Autodesk Inventor part; units mm, degrees
ref_plane "YZ Plane" through (0, 0, 0) normal (1, 0, 0) x (0, 1, 0)
ref_plane "XZ Plane" through (0, 0, 0) normal (0, 1, 0) x (-1, 0, 0)
ref_plane "XY Plane" through (0, 0, 0) normal (0, 0, 1) x (1, 0, 0)
sketch "Sketch1" plane through (0, 0, 0) normal (0, 0, 1) x (1, 0, 0)
  circle A0 centre (-1.3066, -22.8322) radius 2.3
  circle A1 centre (-1.3066, -22.8322) radius 4.5
  circle A2 centre (-1.1075, 27.1674) radius 2.5
  arc A3 (-5.8066, -22.8322) -> (-3.6075, 27.1674) centre (-152.4621, 8.6663) ccw
  arc A4 (1.3925, 27.1674) -> (3.1934, -22.8322) centre (150.0964, 7.4911) ccw
  point P0 (0, 0)
  point P1 (2.8463, -21.0992)
  point P2 (1.3093, 26.5276)
  point P3 (-3.5339, 26.5652)
  point P4 (-5.432, -21.0348)
  dimension "d0" = 4.6
  dimension "d1" = 9
  dimension "d2" = 5
  dimension "d3" = 50
  dimension "d17" = 150
  dimension "d18" = 150
extrude "Extrusion1" add sketch "Sketch1" along normal blind 5 and the other way blind 2
properties part number "gate2"
Part model, mm, in its own coordinate system. Coordinates: 2 decimals unless noted, no trailing zeros. Loops run counter-clockwise (first coordinate to the right, second up) from the corner with the lowest first, then second, coordinate; pieces in that order, holes last. Notation, with made-up numbers: M 2.25,88.25 L 29.25,88.25 A31 ccw 29.25,113.25 Z; hole C 33,-21 d3. An arc over 180 degrees is marked long. Use a Markdown table: item, result. Add a question column.
Q1. Cut at C-C (z = 2). Write the cut outline in (x, y), and give its area (3 significant figures).
Q2. Cut at B-B (x = -0.5). Write the cut outline in (y, z), and give its area (3 significant figures).
Q3. Pin check, flat tips, straight feed: P1, Ø1, axis at x = 1, z = 1.5, coming from the +Y side; P2, Ø3, axis at y = 13, z = 1.5, coming from the -X side; P3, Ø2, axis at y = -18.5, z = 1, coming from the +X side; P4, Ø4, axis at x = -1.31, y = -22.83, coming from the -Z side. Stop position of each tip, or through.
Q4. Cut at A-A (x = -3). Write the cut outline in (y, z), and give its area (3 significant figures).
Q5. Mould opens along Y. For faces 1 (the cylindrical face through (0.186, 2.318, 1.451)), 2 (the flat face through (-1, 2, -2)), 3 (the cylindrical face through (-1.22, -27.33, 1.45)) say: +Y half, -Y half, draft (parallel to the pull), parting line (faces both ways), or undercut.
Q6. Cut at D-D (y = 14.5). Write the cut outline in (x, z).
Q7. Probe L1, parallel to Y at x = -2, z = 3; L2, parallel to Y at x = -0.5, z = 4.5; L3, parallel to X at y = 9, z = 0.5. List the from-to ranges inside material, lowest first.
Worked out:
| question | item | result |
|---|---|---|
| 1 | outline | M -5.43,-21.03 A4.5 ccw long 2.85,-21.1 A150 cw 1.31,26.53 A2.5 ccw long -3.53,26.57 A150 cw Z; hole C -1.31,-22.83 d4.6 |
| 1 | area | 235 mm2 |
| 2 | outline | M -27.26,-2 L -24.99,-2 L -24.99,5 L -27.26,5 Z; M -20.68,-2 L 29.59,-2 L 29.59,5 L -20.68,5 Z |
| 2 | area | 368 mm2 |
| 3 | P1 | stops at y = 29.08 |
| 3 | P2 | stops at x = -2.58 |
| 3 | P3 | stops at x = 2.54 |
| 3 | P4 | passes through |
| 4 | outline | M -27,-2 L -24.39,-2 L -24.39,5 L -27,5 Z; M -21.28,-2 L -4.03,-2 L -4.03,5 L -21.28,5 Z; M 21.36,-2 L 28.8,-2 L 28.8,5 L 21.36,5 Z |
| 4 | area | 191 mm2 |
| 5 | face 1 | undercut |
| 5 | face 2 | draft |
| 5 | face 3 | parting line |
| 6 | outline | M -2.58,-2 L 0.26,-2 L 0.26,5 L -2.58,5 Z |
| 7 | L1 | y = -27.28 to -25.03, -20.64 to 29.5 |
| 7 | L2 | y = -27.26 to -24.99, -20.68 to 29.59 |
| 7 | L3 | x = -2.46 to 0.1 |
